```python
from build123d import *

# Parameters (mm, degrees)
F1_DEPTH = 4


with BuildPart() as f1:
    # F0 (on Top) → F1 (new body)
    with BuildSketch(Plane.XY):
        with BuildLine():
            Line((-36, 71.0140831103), (-44, 71.0140831103))
            add(Edge.make_bspline(
                [(-44, 71.0140831103), (-54.0283164257, 65.6189945034), (-62.2174482843, 57.990161631)],
                knots=[5.235987756, 5.235987756, 5.235987756, 5.4976594153, 5.4976594153, 5.4976594153], degree=2, weights=[1, 0.9914531953, 1]))
            Line((-62.2174482843, 57.990161631), (-49.6600799294, 50.740161631))
            Line((-49.6600799294, 50.740161631), (-73.6600799294, 9.1709422494))
            Line((-73.6600799294, 9.1709422494), (-86.2174482843, 16.4209422494))
            add(Edge.make_bspline(
                [(-86.2174482843, 16.4209422494), (-92.3022663318, -11.319095525), (-78.7223993606, -36.6476383594)],
                knots=[6.0815667198, 6.0815667198, 6.0815667198, 6.7465073975, 6.7465073975, 6.7465073975], degree=2, weights=[1, 0.9452389616, 1]))
            Line((-78.7223993606, -36.6476383594), (-68.4693510334, -26.3945900322))
            Line((-68.4693510334, -26.3945900322), (-34.5282255364, -60.3357155292))
            Line((-34.5282255364, -60.3357155292), (-44.7812738636, -70.5887638564))
            add(Edge.make_bspline(
                [(-44.7812738636, -70.5887638564), (0, -95.2559533934), (44.7812738636, -70.5887638564)],
                knots=[1.0369152893, 1.0369152893, 1.0369152893, 2.1046773643, 2.1046773643, 2.1046773643], degree=2, weights=[1, 0.8608385836, 1]))
            Line((44.7812738636, -70.5887638564), (34.5282255364, -60.3357155292))
            Line((34.5282255364, -60.3357155292), (68.4693510334, -26.3945900322))
            Line((68.4693510334, -26.3945900322), (78.7223993606, -36.6476383594))
            add(Edge.make_bspline(
                [(78.7223993606, -36.6476383594), (92.3022663318, -11.319095525), (86.2174482843, 16.4209422494)],
                knots=[2.6782705633, 2.6782705633, 2.6782705633, 3.343211241, 3.343211241, 3.343211241], degree=2, weights=[1, 0.9452389616, 1]))
            Line((86.2174482843, 16.4209422494), (73.6600799294, 9.1709422494))
            Line((73.6600799294, 9.1709422494), (49.6600799294, 50.740161631))
            Line((49.6600799294, 50.740161631), (62.2174482843, 57.990161631))
            add(Edge.make_bspline(
                [(62.2174482843, 57.990161631), (54.0283164257, 65.6189945034), (44, 71.0140831103)],
                knots=[3.9271185454, 3.9271185454, 3.9271185454, 4.1887902048, 4.1887902048, 4.1887902048], degree=2, weights=[1, 0.9914531953, 1]))
            Line((44, 71.0140831103), (36, 71.0140831103))
            Line((36, 71.0140831103), (36, 62.0140831103))
            Line((36, 62.0140831103), (-36, 62.0140831103))
            Line((-36, 62.0140831103), (-36, 71.0140831103))
        make_face()
    extrude(amount=F1_DEPTH)


solid = f1.part
```
Build history of the part. All positions in model axes, mm. A direction names the side the tool comes from. Round coordinates to 2 decimals unless told otherwise and drop trailing zeros. Loops run counter-clockwise (first coordinate to the right, second up) from the corner with the lowest first, then second, coordinate; pieces in that order, holes last.
Item 1: Two-plate mould, pull along X, no slides. Class faces 1 (the face through (-39.58, -65.39, 1.97)), 2 (the face through (39.727, -65.534, 1.972)), 3 (the face through (-79.851, 12.745, 1.972)): released by +X, released by -X, zero draft, split by the parting line, or undercut.
Item 2: Drill centre lines: line 1 along X through (y, z) = (-36.5, 2.25); line 2 along X through (y, z) = (-71, 1.05); line 3 along Y through (x, z) = (1, 1.7). Where is each one in solid material? Low to high.
Item 3: Pin check, flat tips, straight feed: P1, Ø1.5, axis at y = 48, z = 2, coming from the -X side; P2, Ø2, axis at x = 35, z = 2, coming from the -Y side; P3, Ø2, axis at y = 66.5, z = 1, coming from the +X side; P4, Ø1, axis at x = -67, y = 22, coming from the +Z side. Stop position of each tip, or through.
Item 4: Saw through at B-B (y = 33). List the corners of the cut face in (x, z), then the cut area to 3 significant figures.
Item 5: Saw through at A-A (y = -33.5). State how many separate pieces and enclosed holes the cut face has, then the cut area to 3 significant figures.
Item 6: Saw through at C-C (y = -63). List the corners of the cut face in (x, z).
Item 7: Which spindle directions (+Z, -Z, +X, -X, +Y, -Y) get a long thin tool onto all of the face, cutting with end or side? Do faces 4 (the face through (73.524, -31.449, 1.972)), 5 (the face through (55.851, 54.314, 1.972)), 6 (the face through (-61.49, 30.25, 1.97)), 7 (the face through (36, 67, 2)). Say none if no direction does.
Worked answers:
1. face 1: released by -X
1. face 2: released by +X
1. face 3: undercut
2. line 1: x = -78.8 to -78.57, -58.36 to 58.36, 78.57 to 78.8
2. line 2: x = -44.03 to 44.03
2. line 3: y = -81.99 to 62.01
3. P1: stops at x = -51.68
3. P2: stops at y = -75.63
3. P3: stops at x = 52.94
3. P4: passes through
4. outline: (-59.9, 0) - (59.9, 0) - (59.9, 4) - (-59.9, 4) - close
4. area: 479 mm2
5. separate pieces: 3
5. enclosed holes: 0
5. area: 529 mm2
6. outline: (-37.19, 0) - (37.19, 0) - (37.19, 4) - (-37.19, 4) - close
7. face 4: +Z, -Z, -Y
7. face 5: +Z, -Z, +X
7. face 6: +Z, -Z
7. face 7: +Z, -Z, +Y
